Read the model definition and answer for the solid it produces. Units are mm, in the model's axes. A direction names the side the tool comes from. Coordinates: 2 decimals unless noted, no trailing zeros. Write each loop counter-clockwise with the first axis right and the second up, starting at its lowest first coordinate (ties: lowest second). Pieces come first, ordered by that corner, then holes.
1) The part is cut by section C-C (z = 11.5). Determine the outline of the cut face in (x, y).
2) The part is cut by section B-B (y = 1267). Determine the outline of the cut face in (x, z), then the cut area to 3 significant figures.
3) Find the intervals of material crossed by line 1 (X direction, y = 1724, z = 25.5); line 2 (Y direction, x = 1076.5, z = 53.5), in increasing order.
4) Determine the mould class of faces 1 (the face through (1219.2, 902, 31)), 2 (the face through (0, 902, 31)), 3 (the face through (602, 1765.3, 31)) for opening direction X: +X half, -X half, draft (parallel to the pull), parting line (faces both ways), or undercut.
5) This flat-tipped pin is pushed along its axis until it touches: pin 1 Ø5 at (y, z) = (380, 56.5) entering from -X. Where does it stop, or does it pass through?
6) The part is cut by section A-A (x = 1023). Determine the outline of the cut face in (y, z), then the cut area to 3 significant figures.
7) Which of the six approach directions +Z, -Z, +X, -X, +Y, -Y give full straight-line access (tool end or side, diameter ignored) to faces 4 (the face through (1194, 842, 0)), 5 (the face through (63.5, 902, 31))?
from build123d import *

# Parameters (mm, degrees)
F0_W     = 63.5
F0_H     = 63.5
F1_DEPTH = 1828.8
F2_W     = 63.5
F2_H     = 63.5
F3_DEPTH = 1092.2
F4_W     = 63.5
F4_H     = 63.5
F5_DEPTH = 1828.8
F6_W     = 63.5
F6_H     = 63.5
F7_DEPTH = 1092.2


with BuildPart() as f1:
    # F0 (on Front) → F1 (new body)
    with BuildSketch(Plane.XZ):
        with Locations((31.75, 31.75)):
            Rectangle(F0_W, F0_H)
    extrude(amount=-F1_DEPTH)

    # F2 (on face) → F3 (join)
    with BuildSketch(Plane.YZ.offset(63.5)):
        with Locations((31.75, 31.75)):
            Rectangle(F2_W, F2_H)
    extrude(amount=F3_DEPTH)

    # F4 (on face) → F5 (join)
    with BuildSketch(Plane.XZ):
        with Locations((1187.45, 31.75)):
            Rectangle(F4_W, F4_H)
    extrude(amount=-F5_DEPTH)

    # F6 (on face) → F7 (join)
    with BuildSketch(Plane.YZ.offset(63.5)):
        with Locations((1797.05, 31.75)):
            Rectangle(F6_W, F6_H)
    extrude(amount=F7_DEPTH)


solid = f1.part
Reported:
1. outline: (0, 0) - (1219.2, 0) - (1219.2, 1828.8) - (0, 1828.8) - close; hole (63.5, 63.5) - (1155.7, 63.5) - (1155.7, 1765.3) - (63.5, 1765.3) - close
2. outline: (0, 0) - (63.5, 0) - (63.5, 63.5) - (0, 63.5) - close; (1155.7, 0) - (1219.2, 0) - (1219.2, 63.5) - (1155.7, 63.5) - close
2. area: 8,060 mm2
3. line 1: x = 0 to 63.5, 1155.7 to 1219.2
3. line 2: y = 0 to 63.5, 1765.3 to 1828.8
4. face 1: +X half
4. face 2: -X half
4. face 3: undercut
5. pin 1: stops at x = 0
6. outline: (0, 0) - (63.5, 0) - (63.5, 63.5) - (0, 63.5) - close; (1765.3, 0) - (1828.8, 0) - (1828.8, 63.5) - (1765.3, 63.5) - close
6. area: 8,060 mm2
7. face 4: -Z, +X, -X, +Y, -Y
7. face 5: +Z, -Z
